Check sheet for the modelled part. Datum: model origin and axes. Units: mm. Give positions to 0.01 mm unless a question says otherwise; leave off trailing zeros. Write each loop counter-clockwise with the first axis right and the second up, starting at its lowest first coordinate (ties: lowest second). Pieces come first, ordered by that corner, then holes. Notation, with made-up numbers: (-36, 21) - (-7, 21) arc R17 ccw to (-7, 26) - close; hole circle Ø9 at (-27, -35.75). An arc over 180 degrees is marked (long way). Return JSON: item names as keys, results as strings. Group by question number.
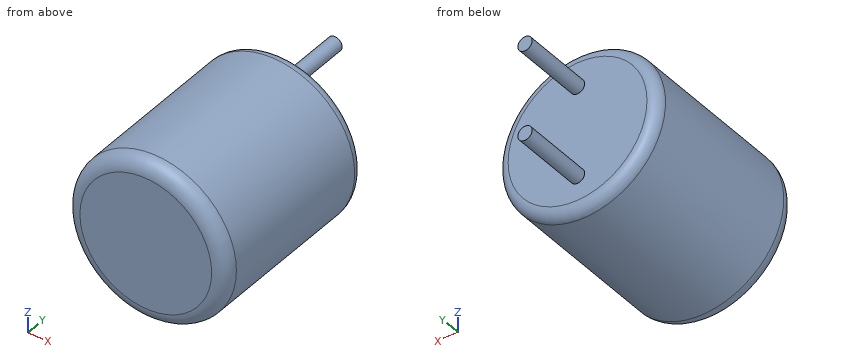
Autodesk Fusion 360 part; units mm, degrees
sketch "Sketch1" plane through (0, 0, 0) normal (0, 1, 0) x (1, 0, 0)
  circle A0 centre (0, 0) radius 2.25
  dimension "d1" = 4.5
extrude "Extrude1" add sketch "Sketch1" along normal blind 5.2
sketch "Sketch2" plane through (0, 5.2, 0) normal (0, 1, 0) x (-1, 0, 0)
  circle A0 centre (0, 0) radius 2.25
  line L0 (0, 0) -> (0, -1.27)
  circle A1 centre (0, -1.27) radius 0.2
  line L1 (0, 0) -> (-0.6583, 0) construction
  circle A2 centre (0, 1.27) radius 0.2
  dimension "d4" = 1.27
  dimension "d6" = 0.4
extrude "Extrude2" add sketch "Sketch2" along normal blind 2 contours A1 | A2
fillet "Fillet1" radius 0.4 1 edges at (-2.0977, 0, 0.8136)
fillet "Fillet2" radius 0.3 1 edges at (-2.0977, 5.2, 0.8136)
sketch "Sketch3" plane through (0, 0, 0) normal (0, 0, 1) x (1, 0, 0)
equation "d4 = ( 2.54 / 2 ) * 1 mm"
Item 1: Section check D-D on y = 4.5. Record the cut outline in (x, z), plus the area to 3 significant figures.
Item 2: Material ranges on line 1 along Y through (x, z) = (0.2, 0.05); line 2 along X through (y, z) = (5.5, 1.25); line 3 along Z through (x, y) = (0.8, 0.5), recorded low to high. Write a range as from..to.
Item 3: Section check B-B on y = 5.75. Record the cut outline in (x, z), plus the area to 3 significant figures.
Item 4: Depth check by flat-ended pin: pin 1 (1 mm diameter, centred on y = 1, z = -1.5, fed in from +X); pin 2 (1 mm diameter, centred on y = 5.5, z = 1, fed in from +X). Enter the tip coordinate at first touch or a pass-through.
Item 5: Section check A-A on z = 0. Record the cut outline in (x, y).
Item 6: Section check C-C on x = 0. Record the cut outline in (y, z).
Reply:
{
 "1": {"outline": "circle Ø4.5 at (0, 0)", "area": "15.9 mm²"},
 "2": {"line 1": "0..5.2", "line 2": "-0.2..0.2", "line 3": "-2.1..2.1"},
 "3": {"outline": "circle Ø0.4 at (0, -1.27); circle Ø0.4 at (0, 1.27)", "area": "0.251 mm²"},
 "4": {"pin 1": "x = 2.02", "pin 2": "x = 2.07"},
 "5": {"outline": "(-2.25, 0.4) arc R0.4 ccw to (-1.85, 0) - (1.85, 0) arc R0.4 ccw to (2.25, 0.4) - (2.25, 4.9) arc R0.3 ccw to (1.95, 5.2) - (-1.95, 5.2) arc R0.3 ccw to (-2.25, 4.9) - close"},
 "6": {"outline": "(0, -1.85) arc R0.4 ccw to (0.4, -2.25) - (4.9, -2.25) arc R0.3 ccw to (5.2, -1.95) - (5.2, -1.47) - (7.2, -1.47) - (7.2, -1.07) - (5.2, -1.07) - (5.2, 1.07) - (7.2, 1.07) - (7.2, 1.47) - (5.2, 1.47) - (5.2, 1.95) arc R0.3 ccw to (4.9, 2.25) - (0.4, 2.25) arc R0.4 ccw to (0, 1.85) - close"}
}
